```python
from build123d import *

# Parameters (mm, degrees)
SKETCH1_R           = 6.5024
BOSS_EXTRUDE1_DEPTH = 33.401
SKETCH2_R           = 4.3688
CUT_EXTRUDE1_DEPTH  = 33.401


with BuildPart() as part:
    # Sketch1 → Boss-Extrude1 (new body)
    with BuildSketch(Plane(origin=(0, 0, 0), x_dir=(1, 0, 0), z_dir=(0, 1, 0))):
        with Locations(Location((0, 0, 0), (0, 0, 270))):
            Circle(SKETCH1_R)
    extrude(amount=BOSS_EXTRUDE1_DEPTH)

    # Sketch2 → Cut-Extrude1 (cut)
    with BuildSketch(Plane(origin=(0, 0, 0), x_dir=(1, 0, 0), z_dir=(0, 1, 0))):
        with Locations(Location((0, 0, 0), (0, 0, 270))):
            Circle(SKETCH2_R)
    extrude(amount=CUT_EXTRUDE1_DEPTH, mode=Mode.SUBTRACT)

    # Sketch3 → Revolve2 (revolve)
    with BuildSketch(Plane.XY, mode=Mode.PRIVATE) as revolve2_sk:
        Polygon((6.5024, 33.401), (8.0518, 33.401), (8.4328, 29.2354), (6.5024, 29.2354), align=None)
    revolve(revolve2_sk.sketch.rotate(Axis((0, 33.401, 0), (0, -1, 0)), 90), axis=Axis((0, 33.401, 0), (0, -1, 0)))


solid = part.part
```
Source: CAD feature listing. Evaluate the final solid. Frame: model axes, mm. Coordinates: 2 decimals unless noted, no trailing zeros. Write each loop counter-clockwise with the first axis right and the second up, starting at its lowest first coordinate (ties: lowest second). Pieces come first, ordered by that corner, then holes. Notation, with made-up numbers: (35.25, 67) - (82.25, 67) arc R13 ccw to (82.25, 85) - close; hole circle Ø3 at (65, -27). An arc over 180 degrees is marked (long way). Answer as a JSON object with one key per item and string values.
Q1. Draft query along Z for faces 1 (the cylindrical face through (1.312, 16.467, 4.167)), 2 (the flat face through (3.5, 33.401, -3.5)), 3 (the conical face through (7.24, 32.215, 3.765)). Return one class per face: released by +Z, released by -Z, zero draft, split by the parting line, or undercut.
Ans:
{"face 1": "undercut", "face 2": "zero draft", "face 3": "split by the parting line"}
Q2. Section query B-B, the plane x = 0. Output: boundary loops of the cut face in (y, z).
Ans:
{"outline": "(0, -6.5) - (29.24, -6.5) - (29.24, -8.43) - (33.4, -8.05) - (33.4, -4.37) - (0, -4.37) - close; (0, 4.37) - (33.4, 4.37) - (33.4, 8.05) - (29.24, 8.43) - (29.24, 6.5) - (0, 6.5) - close"}
Q3. Section query C-C, the plane y = 6. Output: boundary loops of the cut face in (x, z).
Ans:
{"outline": "circle Ø13 at (0, 0); hole circle Ø8.74 at (0, 0)"}
Q4. First-contact query: pin 1 Ø8 at (y, z) = (4.5, 0.5) entering from +X; pin 2 Ø1 at (x, y) = (1.5, 11.5) entering from -Z; pin 3 Ø6 at (y, z) = (23.5, -1.5) entering from -X. Flat tips, straight axial feed; report the tip coordinate or a pass-through.
Ans:
{"pin 1": "stops at x = 6.5", "pin 2": "stops at z = -6.43", "pin 3": "stops at x = -6.5"}
Q5. Section query A-A, the plane z = 0. Output: boundary loops of the cut face in (x, y).
Ans:
{"outline": "(-8.43, 29.24) - (-6.5, 29.24) - (-6.5, 0) - (-4.37, 0) - (-4.37, 33.4) - (-8.05, 33.4) - close; (4.37, 0) - (6.5, 0) - (6.5, 29.24) - (8.43, 29.24) - (8.05, 33.4) - (4.37, 33.4) - close"}
Q6. Section query D-D, the plane y = 30. Output: boundary loops of the cut face in (x, z), plus the area to 3 significant figures.
Ans:
{"outline": "circle Ø16.73 at (0, 0); hole circle Ø8.74 at (0, 0)", "area": "160 mm2"}
Q7. Material intervals for line 1 (X direction, y = 16, z = 0); line 2 (Y direction, x = -6.25, z = -2.25); line 3 (X direction, y = 32, z = 3.25), sorted ascending. Write a range as [from, to].
Ans:
{"line 1": "x = [-6.5, -4.37], [4.37, 6.5]", "line 2": "y = [29.24, 33.4]", "line 3": "x = [-7.51, -2.92], [2.92, 7.51]"}
